Model file for the job. Use its own axes, mm. A direction names the side the tool comes from. Coordinates: 2 decimals unless noted, no trailing zeros. Order: outer loops, then holes, each group sorted by start corner. A loop starts at its lowest first (then second) coordinate and runs counter-clockwise, first axis right, second up.
from build123d import *

# Parameters (mm, degrees)
ESQUISSE1_W      = 4.949747468
ESQUISSE1_H      = 4.949747468
EXTRUSION1_DEPTH = 11
ESQUISSE2_R      = 5.5
EXTRUSION2_DEPTH = 1
ESQUISSE3_R      = 1.5
EXTRUSION3_DEPTH = 15.300349646
CONG_1_R         = 0.5


with BuildPart() as part:
    # Esquisse1 → Extrusion1 (new body)
    with BuildSketch(Plane.XY):
        Rectangle(ESQUISSE1_W, ESQUISSE1_H)
    extrude(amount=EXTRUSION1_DEPTH)

    # Esquisse2 → Extrusion2 (add)
    with BuildSketch(Plane.XY.offset(11)):
        Circle(ESQUISSE2_R)
    extrude(amount=EXTRUSION2_DEPTH)

    # Esquisse3 → Extrusion3 (cut, through all)
    with BuildSketch(Plane.XY.offset(12)):
        Circle(ESQUISSE3_R)
    extrude(amount=-EXTRUSION3_DEPTH, mode=Mode.SUBTRACT)

    # Congé1
    cong_1_edges = [part.edges().sort_by_distance(p)[0] for p in [
        (0, 2.474873734, 0),
        (2.474873734, 0, 0),
        (0, -2.474873734, 0),
        (-2.474873734, 0, 0),
        (-2.474873734, 2.474873734, 5.5),
        (2.474873734, 2.474873734, 5.5),
        (2.474873734, -2.474873734, 5.5),
        (-2.474873734, -2.474873734, 5.5),
    ]]
    fillet(cong_1_edges, radius=CONG_1_R)


solid = part.part
Q1. Drop flat-ended pins along their axis: P1, Ø1.2, axis at x = 0.5, z = 7.5, coming from the -Y side; P2, Ø4.5, axis at y = -0.5, z = 7.5, coming from the +X side; P3, Ø1, axis at x = 4.5, y = 3, coming from the -Z side. Give the stop position or say it passes through.
Established:
P1: stops at y = -2.47
P2: stops at x = 2.47
P3: stops at z = 11
Q2. Mould opens along X. For faces 4 (the face through (2.475, 0, 6)), 5 (the face through (-1.5, 0.07, 6.08)), 6 (the face through (0, 2.475, 6)) say: pulls with the +X half, pulls with the -X half, needs draft (parallel to the pull), parting line crosses it, or undercut.
Established:
face 4: pulls with the +X half
face 5: undercut
face 6: needs draft
Q3. Cut at A-A, the plane z = 10. List the corners of the cut face in (x, y), plus the area to 3 significant figures.
Established:
outline: (-2.47, -1.97) arc R0.5 ccw to (-1.97, -2.47) - (1.97, -2.47) arc R0.5 ccw to (2.47, -1.97) - (2.47, 1.97) arc R0.5 ccw to (1.97, 2.47) - (-1.97, 2.47) arc R0.5 ccw to (-2.47, 1.97) - close; hole circle Ø3 at (0, 0)
area: 17.2 mm2
Q4. Which spindle directions (+Z, -Z, +X, -X, +Y, -Y) get a long thin tool onto all of the face, cutting with end or side? Do faces 1 (the face through (0, -2.475, 6)), 2 (the face through (-3, 0, 11)), 3 (the face through (-2.475, 0, 6)). Say none if no direction does.
Established:
face 1: -Z, +X, -X, -Y
face 2: -Z
face 3: -Z, -X, +Y, -Y
Q5. Cut at D-D, the plane y = -1.75. List the corners of the cut face in (x, z), plus the area to 3 significant figures.
Established:
outline: (-5.21, 11) - (-2.47, 11) - (-2.47, 0.5) arc R0.5 ccw to (-1.97, 0) - (1.97, 0) arc R0.5 ccw to (2.47, 0.5) - (2.47, 11) - (5.21, 11) - (5.21, 12) - (-5.21, 12) - close
area: 64.8 mm2
Q6. Probe line 1 (Y direction, x = 0, z = 8.5); line 2 (Z direction, x = 3.5, y = -1); line 3 (X direction, y = -1.25, z = 8.75). List the from-to ranges inside material, lowest first.
Established:
line 1: y = -2.47 to -1.5, 1.5 to 2.47
line 2: z = 11 to 12
line 3: x = -2.47 to -0.83, 0.83 to 2.47
Q7. Cut at B-B, the plane x = 0. List the corners of the cut face in (y, z), plus the area to 3 significant figures.
Established:
outline: (-5.5, 11) - (-2.47, 11) - (-2.47, 0.5) arc R0.5 ccw to (-1.97, 0) - (-1.5, 0) - (-1.5, 12) - (-5.5, 12) - close; (1.5, 0) - (1.97, 0) arc R0.5 ccw to (2.47, 0.5) - (2.47, 11) - (5.5, 11) - (5.5, 12) - (1.5, 12) - close
area: 29.3 mm2
